The listing builds one solid part. Answer for the finished solid, in the listing's coordinates (mm). A direction names the side the tool comes from. Give positions to 0.01 mm unless a question says otherwise; leave off trailing zeros. Order: outer loops, then holes, each group sorted by start corner. A loop starts at its lowest first (then second) coordinate and runs counter-clockwise, first axis right, second up. Notation, with made-up numbers: (47, 61) - (81, 61) arc R22 ccw to (81, 70) - close; hole circle Ø6 at (-4.5, 80). An arc over 180 degrees is marked (long way). Answer as a JSON object with one key per item and string values. Group by question number.
Q1. A cutting plane is placed at A-A, the plane y = 12. Give the vertices of the cut face in (x, z), and give its area (3 significant figures).
Q2. For faces 1 (the face through (10, 2, -22)), 2 (the face through (86, 8, -2)), 3 (the face through (47, 9, -39)), determine the directions among +Z, -Z, +X, -X, +Y, -Y from which every point of the face is accessible in a straight line to the end or side of a thin tool.
Q3. Given pin 1 (2 mm diameter, centred on y = 2, z = -20.5, fed in from -X); pin 2 (2 mm diameter, centred on x = 12, z = -27.2, fed in from +Y); pin 3 (4.5 mm diameter, centred on x = 10, z = -6.5, fed in from +Y); pin 4 (0.9 mm diameter, centred on x = 9.5, z = -15.5, fed in from +Y), each flat-ended and moving along its own axis, determine where each tip first touches the part or whether it passes through.
Q4. A cutting plane is placed at C-C, the plane z = -6.5. Give the vertices of the cut face in (x, y).
Q5. The mould has two halves that part along Z. Classify faces 4 (the face through (43.89, 1.5, -36.68)), 5 (the face through (92.43, 6.9, -42.4)), 6 (the face through (92.4, 6.9, -0.57)): released by +Z, released by -Z, zero draft, split by the parting line, or undercut.
Q6. A cutting plane is placed at D-D, the plane x = 59. Give the vertices of the cut face in (y, z).
Q7. A cutting plane is placed at B-B, the plane x = 70.2. Give the vertices of the cut face in (y, z).
Q8. Consider line 1 (X direction, y = 6.25, z = -27.2); line 2 (X direction, y = 7.5, z = -14); line 3 (Z direction, x = 59, y = 3). Determine where each line is inside the solid, lowest interval first.
from build123d import *
from OCP.BRepFilletAPI import BRepFilletAPI_MakeChamfer

# Parameters (mm, degrees)
SKETCH1_W               = 93
SKETCH1_H               = 43
SKETCH1_R               = 1.4
SKETCH1_W_2             = 51
SKETCH1_H_2             = 21
SKETCH1_W_3             = 21
SKETCH1_H_3             = 34
BOSS_EXTRUDE1_DEPTH     = 4
BOSS_EXTRUDE2_OUTLINE_W = 53.222222222
BOSS_EXTRUDE2_OUTLINE_H = 21
BOSS_EXTRUDE2_OUTLINE_R = 1.4
BOSS_EXTRUDE2_DEPTH     = 8
SKETCH1_4_W             = 21
SKETCH1_4_H             = 34
SKETCH1_4_R             = 1.5
BOSS_EXTRUDE3_DEPTH     = 4
CHAMFER1_SIZE           = 0.6
CHAMFER1_SIZE2          = 0.960200717
SKETCH2_W               = 10
SKETCH2_H               = 10
CUT_EXTRUDE1_DEPTH      = 4
BOSS_EXTRUDE4_DEPTH     = 10
FILLET1_R               = 2
SKETCH5_W               = 5
SKETCH5_H               = 4
CUT_EXTRUDE3_DEPTH      = 6


# Read off the part's stored shape, not the designer's step: Boss-Extrude2
with BuildPart() as part:
    # Sketch1 → Boss-Extrude1 (new body)
    with BuildSketch(Plane(origin=(0, 0, 0), x_dir=(1, 0, 0), z_dir=(0, 1, 0))):
        with Locations((46.5, 21.5)):
            Rectangle(SKETCH1_W, SKETCH1_H)
        with Locations(Location((10, 36.5, 0), (0, 0, 270))):
            Circle(SKETCH1_R, mode=Mode.SUBTRACT)
        with Locations(Location((42.5, 36.5, 0), (0, 0, 270))):
            Circle(SKETCH1_R, mode=Mode.SUBTRACT)
        with Locations(Location((42.5, 6.5, 0), (0, 0, 270))):
            Circle(SKETCH1_R, mode=Mode.SUBTRACT)
        with Locations(Location((10, 6.5, 0), (0, 0, 270))):
            Circle(SKETCH1_R, mode=Mode.SUBTRACT)
        with Locations((35.5, 21.5)):
            Rectangle(SKETCH1_W_2, SKETCH1_H_2, mode=Mode.SUBTRACT)
        with Locations((77.5, 21.5)):
            Rectangle(SKETCH1_W_3, SKETCH1_H_3, mode=Mode.SUBTRACT)
    extrude(amount=BOSS_EXTRUDE1_DEPTH)

    # Boss-Extrude2 outline → Boss-Extrude2 (add)
    with BuildSketch(Plane(origin=(0, 0, 0), x_dir=(1, 0, 0), z_dir=(0, 1, 0))):
        with Locations((34.611111111, 21.5)):
            Rectangle(BOSS_EXTRUDE2_OUTLINE_W, BOSS_EXTRUDE2_OUTLINE_H)
        with Locations((10.222222222, 15.8)):
            Circle(BOSS_EXTRUDE2_OUTLINE_R, mode=Mode.SUBTRACT)
        with Locations((12, 27.2)):
            Circle(BOSS_EXTRUDE2_OUTLINE_R, mode=Mode.SUBTRACT)
        with Locations((59, 27.2)):
            Circle(BOSS_EXTRUDE2_OUTLINE_R, mode=Mode.SUBTRACT)
        with Locations((59, 15.8)):
            Circle(BOSS_EXTRUDE2_OUTLINE_R, mode=Mode.SUBTRACT)
    extrude(amount=BOSS_EXTRUDE2_DEPTH)

    # Sketch1<4> → Boss-Extrude3 (add)
    with BuildSketch(Plane(origin=(0, 0, 0), x_dir=(1, 0, 0), z_dir=(0, 1, 0))):
        with Locations((77.5, 21.5)):
            Rectangle(SKETCH1_4_W, SKETCH1_4_H)
        with Locations(Location((70.2, 34.2, 0), (0, 0, 270))):
            Circle(SKETCH1_4_R, mode=Mode.SUBTRACT)
        with Locations(Location((84.8, 34.2, 0), (0, 0, 270))):
            Circle(SKETCH1_4_R, mode=Mode.SUBTRACT)
    extrude(amount=BOSS_EXTRUDE3_DEPTH)

    # Chamfer1: one chamfer whose edges measure the first distance from different faces: ONE call of the kernel's chamfer builder (chamfer() names one face for all edges)
    chamfer1_edges_1 = [part.edges().sort_by_distance(p)[0] for p in [
        (42.5, 4, -7.9),
    ]]
    chamfer1_side_1 = [part.faces().sort_by_distance(p)[0] for p in [
        (42.5, 2, -7.9),
    ]]
    chamfer1_edges_2 = [part.edges().sort_by_distance(p)[0] for p in [
        (42.5, 4, -37.9),
        (10, 4, -37.9),
    ]]
    chamfer1_side_2 = [part.faces().sort_by_distance(p)[0] for p in [
        (46.5, 4, -1.024597482),
    ]]
    chamfer1_edges_3 = [part.edges().sort_by_distance(p)[0] for p in [
        (10, 4, -7.9),
    ]]
    chamfer1_side_3 = [part.faces().sort_by_distance(p)[0] for p in [
        (10, 2, -7.9),
    ]]
    chamfer1 = BRepFilletAPI_MakeChamfer(part.part.solid().wrapped)
    for e in chamfer1_edges_1:
        chamfer1.Add(CHAMFER1_SIZE, CHAMFER1_SIZE2, e.wrapped, chamfer1_side_1[0].wrapped)  # the first distance lies on this face
    for e in chamfer1_edges_2:
        chamfer1.Add(CHAMFER1_SIZE, CHAMFER1_SIZE2, e.wrapped, chamfer1_side_2[0].wrapped)  # the first distance lies on this face
    for e in chamfer1_edges_3:
        chamfer1.Add(CHAMFER1_SIZE, CHAMFER1_SIZE2, e.wrapped, chamfer1_side_3[0].wrapped)  # the first distance lies on this face
    add(Compound.cast(chamfer1.Shape()), mode=Mode.REPLACE)

    # Sketch2 → Cut-Extrude1 (cut)
    with BuildSketch(Plane.XZ):
        with Locations((5, -21.5)):
            Rectangle(SKETCH2_W, SKETCH2_H)
    extrude(amount=-CUT_EXTRUDE1_DEPTH, mode=Mode.SUBTRACT)

    # Sketch3 → Boss-Extrude4 (add)
    with BuildSketch(Plane(origin=(0, 4, 0), x_dir=(1, 0, 0), z_dir=(0, 1, 0))):
        Polygon((4, 39), (4, 26.5), (0, 26.5), (0, 43), (93, 43), (93, 0), (0, 0), (0, 16.5), (4, 16.5), (4, 4), (89, 4), (89, 39), align=None)
    extrude(amount=BOSS_EXTRUDE4_DEPTH)

    # Fillet1
    fillet1_edges = [part.edges().sort_by_distance(p)[0] for p in [
        (0, 7, 0),
        (0, 7, -43),
        (93, 7, -43),
        (93, 7, 0),
    ]]
    fillet(fillet1_edges, radius=FILLET1_R)

    # Sketch5 → Cut-Extrude3 (cut)
    with BuildSketch(Plane(origin=(0, 14, 0), x_dir=(1, 0, 0), z_dir=(0, 1, 0))):
        with Locations((86.5, 2)):
            Rectangle(SKETCH5_W, SKETCH5_H)
    extrude(amount=-CUT_EXTRUDE3_DEPTH, mode=Mode.SUBTRACT)


solid = part.part
Reply:
{
 "1": {"outline": "(0, -41) arc R2 ccw to (2, -43) - (91, -43) arc R2 ccw to (93, -41) - (93, -2) arc R2 ccw to (91, 0) - (89, 0) - (89, -39) - (4, -39) - (4, -26.5) - (0, -26.5) - close; (0, -16.5) - (4, -16.5) - (4, -4) - (84, -4) - (84, 0) - (2, 0) arc R2 ccw to (0, -2) - close", "area": "961 mm^2"},
 "2": {"face 1": "-X, -Y", "face 2": "+Z, +Y", "face 3": "+Y"},
 "3": {"pin 1": "stops at x = 10", "pin 2": "passes through", "pin 3": "stops at y = 3.93", "pin 4": "stops at y = 4"},
 "4": {"outline": "(0, 0) - (8.6, 0) - (8.6, 3.4) - (7.64, 4) - (4, 4) - (4, 14) - (0, 14) - close; (11.4, 0) - (41.1, 0) - (41.1, 3.4) - (40.14, 4) - (12.36, 4) - (11.4, 3.4) - close; (43.9, 0) - (93, 0) - (93, 14) - (89, 14) - (89, 4) - (44.86, 4) - (43.9, 3.4) - close"},
 "5": {"face 4": "undercut", "face 5": "released by -Z", "face 6": "released by +Z"},
 "6": {"outline": "(0, -43) - (14, -43) - (14, -39) - (4, -39) - (4, -32) - (8, -32) - (8, -28.6) - (0, -28.6) - close; (0, -25.8) - (8, -25.8) - (8, -17.2) - (0, -17.2) - close; (0, -14.4) - (8, -14.4) - (8, -11) - (4, -11) - (4, -4) - (14, -4) - (14, 0) - (0, 0) - close"},
 "7": {"outline": "(0, -43) - (14, -43) - (14, -39) - (4, -39) - (4, -35.7) - (0, -35.7) - close; (0, -32.7) - (4, -32.7) - (4, -4) - (14, -4) - (14, 0) - (0, 0) - close"},
 "8": {"line 1": "x = 0 to 4, 8 to 10.6, 13.4 to 57.6, 60.4 to 61.22, 89 to 93", "line 2": "x = 0 to 4, 8 to 61.22, 89 to 93", "line 3": "z = -43 to -28.6, -25.8 to -17.2, -14.4 to 0"}
}
